Geometry check sheet. Reference: the model listing, model coordinates, mm. A direction names the side the tool comes from. Round coordinates to 2 decimals unless told otherwise and drop trailing zeros. Order: outer loops, then holes, each group sorted by start corner. A loop starts at its lowest first (then second) coordinate and runs counter-clockwise, first axis right, second up.
(1) Go/stop test with flat-tipped pins: pin 1 (6 mm diameter, centred on x = -57.5, z = -4, fed in from -Y); pin 2 (0.6 mm diameter, centred on x = -33, y = 32, fed in from +Z); pin 3 (4 mm diameter, centred on x = -49, y = 16, fed in from +Z); pin 4 (5 mm diameter, centred on y = 10, z = 9.5, fed in from +X). Record where each tip stops, or that it passes through.
(2) Set-up check for faces 4 (the face through (-34.161, 27, -15)), 5 (the face through (-33, 27, -12.512)), 6 (the face through (-32.76, 27.12, -21.94)): record each of +Z, -Z, +X, -X, +Y, -Y from which the full face is reachable in a straight line by a thin tool's end or side.
(3) Sectioned sample at A-A (z = -15). Record the boundary of the cut face in (x, y), plus the area to 3 significant figures.
(4) Sectioned sample at B-B (y = 27.5). Record the boundary of the cut face in (x, z).
(5) Sectioned sample at C-C (x = -43.75). Record the boundary of the cut face in (y, z), plus the area to 3 significant figures.
(6) Release check for a two-part mould opening along X. For faces 1 (the face through (-59.5, 55, -6.9)), 2 (the face through (-60.6, 27.1, -21.9)), 3 (the face through (-50.78, 25.58, -21.53)) record: +X half, -X half, draft (parallel to the pull), parting line (faces both ways), or undercut.
(7) Material ranges on line 1 along X through (y, z) = (9.5, -13); line 2 along Z through (x, y) = (-47.5, 50); line 3 along Z through (x, y) = (-60.7, 27.5), recorded low to high.
(8) Sectioned sample at D-D (y = 6). Record the boundary of the cut face in (x, z), plus the area to 3 significant figures.
from build123d import *

# Parameters (mm, degrees)
BOSS_EXTRUDE1_DEPTH              = 55
M10X1_0_TAPPED_HOLE2_D           = 9
M10X1_0_TAPPED_HOLE2_DEPTH       = 23
M10X1_0_TAPPED_HOLE2_CBORE_D     = 10
M10X1_0_TAPPED_HOLE2_CBORE_DEPTH = 20
M10X1_0_TAPPED_HOLE2_TIP         = 2.703872786
M10X1_0_TAPPED_HOLE1_D           = 9
M10X1_0_TAPPED_HOLE1_DEPTH       = 23
M10X1_0_TAPPED_HOLE1_CBORE_D     = 10
M10X1_0_TAPPED_HOLE1_CBORE_DEPTH = 20
M10X1_0_TAPPED_HOLE1_TIP         = 2.703872786


with BuildPart() as part:
    # Sketch1 → Boss-Extrude1 (new body)
    with BuildSketch(Plane(origin=(0, 0, 0), x_dir=(1, 0, 0), z_dir=(0, 1, 0))):
        with BuildLine():
            Line((-61.161397451, -27.487824391), (-61.161397451, 20.512175609))
            ThreePointArc((-61.161397451, 20.512175609), (-60.575611013, 21.926389171), (-59.161397451, 22.512175609))
            Line((-59.161397451, 22.512175609), (-34.161397451, 22.512175609))
            ThreePointArc((-34.161397451, 22.512175609), (-32.747183888, 21.926389171), (-32.161397451, 20.512175609))
            Line((-32.161397451, 20.512175609), (-32.161397451, 12.512175609))
            Line((-32.161397451, 12.512175609), (-34.161397451, 12.512175609))
            Line((-34.161397451, 12.512175609), (-34.161397451, 18.512175609))
            ThreePointArc((-34.161397451, 18.512175609), (-34.747183888, 19.926389171), (-36.161397451, 20.512175609))
            Line((-36.161397451, 20.512175609), (-57.161397451, 20.512175609))
            ThreePointArc((-57.161397451, 20.512175609), (-58.575611013, 19.926389171), (-59.161397451, 18.512175609))
            Line((-59.161397451, 18.512175609), (-59.161397451, -27.487824391))
            Line((-59.161397451, -27.487824391), (-61.161397451, -27.487824391))
        make_face()
    extrude(amount=BOSS_EXTRUDE1_DEPTH)

    # M10x1.0 Tapped Hole2
    with Locations(Plane(origin=(-46.161397451, 27.5, -22.512175609), x_dir=(-1, 0, 0), z_dir=(0, 0, -1))):
        with Locations((0, 0)):
            CounterBoreHole(M10X1_0_TAPPED_HOLE2_D / 2, M10X1_0_TAPPED_HOLE2_CBORE_D / 2, M10X1_0_TAPPED_HOLE2_CBORE_DEPTH, depth=M10X1_0_TAPPED_HOLE2_DEPTH)
            with Locations((0, 0, -(M10X1_0_TAPPED_HOLE2_DEPTH + M10X1_0_TAPPED_HOLE2_TIP / 2))):  # 118° drill point
                Cone(0, M10X1_0_TAPPED_HOLE2_D / 2, M10X1_0_TAPPED_HOLE2_TIP, mode=Mode.SUBTRACT)

    # M10x1.0 Tapped Hole1
    with Locations(Plane(origin=(-61.161397451, 27.5, 7.487824391), x_dir=(0, 0, -1), z_dir=(-1, 0, 0))):
        with Locations((0, 0)):
            CounterBoreHole(M10X1_0_TAPPED_HOLE1_D / 2, M10X1_0_TAPPED_HOLE1_CBORE_D / 2, M10X1_0_TAPPED_HOLE1_CBORE_DEPTH, depth=M10X1_0_TAPPED_HOLE1_DEPTH)
            with Locations((0, 0, -(M10X1_0_TAPPED_HOLE1_DEPTH + M10X1_0_TAPPED_HOLE1_TIP / 2))):  # 118° drill point
                Cone(0, M10X1_0_TAPPED_HOLE1_D / 2, M10X1_0_TAPPED_HOLE1_TIP, mode=Mode.SUBTRACT)


solid = part.part
Answer below:
1. pin 1: stops at y = 0
1. pin 2: stops at z = -12.51
1. pin 3: stops at z = -20.51
1. pin 4: stops at x = -59.16
2. face 4: +Z, +Y, -Y
2. face 5: +Z, +X, +Y, -Y
2. face 6: -Z, +X, +Y, -Y
3. outline: (-61.16, 0) - (-59.16, 0) - (-59.16, 55) - (-61.16, 55) - close; (-34.16, 0) - (-32.16, 0) - (-32.16, 55) - (-34.16, 55) - close
3. area: 220 mm2
4. outline: (-61.16, -20.51) arc R2 ccw to (-59.16, -22.51) - (-51.16, -22.51) - (-51.16, -20.51) - (-57.16, -20.51) arc R2 cw to (-59.16, -18.51) - (-59.16, 2.49) - (-61.16, 2.49) - close; (-61.16, 12.49) - (-59.16, 12.49) - (-59.16, 27.49) - (-61.16, 27.49) - close; (-41.16, -22.51) - (-34.16, -22.51) arc R2 ccw to (-32.16, -20.51) - (-32.16, -12.51) - (-34.16, -12.51) - (-34.16, -18.51) arc R2 cw to (-36.16, -20.51) - (-41.16, -20.51) - close
5. outline: (0, -22.51) - (23.12, -22.51) - (23.12, -20.51) - (0, -20.51) - close; (31.88, -22.51) - (55, -22.51) - (55, -20.51) - (31.88, -20.51) - close
5. area: 92.5 mm2
6. face 1: draft
6. face 2: -X half
6. face 3: undercut
7. line 1: x = -61.16 to -59.16, -34.16 to -32.16
7. line 2: z = -22.51 to -20.51
7. line 3: z = -21.79 to 2.49, 12.49 to 27.49
8. outline: (-61.16, -20.51) arc R2 ccw to (-59.16, -22.51) - (-34.16, -22.51) arc R2 ccw to (-32.16, -20.51) - (-32.16, -12.51) - (-34.16, -12.51) - (-34.16, -18.51) arc R2 cw to (-36.16, -20.51) - (-57.16, -20.51) arc R2 cw to (-59.16, -18.51) - (-59.16, 27.49) - (-61.16, 27.49) - close
8. area: 170 mm2
